Verification items for the finished model (mm, model axes). A direction names the side the tool comes from. Give positions to 0.01 mm unless a question says otherwise; leave off trailing zeros. Write each loop counter-clockwise with the first axis right and the second up, starting at its lowest first coordinate (ties: lowest second). Pieces come first, ordered by that corner, then holes. Notation, with made-up numbers: (-25, 81.5) -> (-9, 81.5) arc R16 cw to (-9, 106.5) -> close; hole circle Ø9 at (28, 69.25). An arc over 180 degrees is marked (long way). Write item = value, one per line.
from build123d import *

# Parameters (mm, degrees)
SKETCH1_W           = 215
SKETCH1_H           = 88
SKETCH1_R           = 1.75
BOSS_EXTRUDE1_DEPTH = 4
FILLET1_R           = 15
FILLET2_R           = 40
BOSS_EXTRUDE2_DEPTH = 160
SKETCH3_R           = 1.6
CUT_EXTRUDE1_DEPTH  = 4


with BuildPart() as part:
    # Sketch1 → Boss-Extrude1 (new body)
    with BuildSketch(Plane.XY):
        with Locations((-8, 0)):
            Rectangle(SKETCH1_W, SKETCH1_H)
        with Locations((-26.5, 20)):
            Circle(SKETCH1_R, mode=Mode.SUBTRACT)
        with Locations((26.5, 20)):
            Circle(SKETCH1_R, mode=Mode.SUBTRACT)
        with Locations((-26.5, -20)):
            Circle(SKETCH1_R, mode=Mode.SUBTRACT)
        with Locations((26.5, -20)):
            Circle(SKETCH1_R, mode=Mode.SUBTRACT)
        with Locations((0, 20)):
            Circle(SKETCH1_R, mode=Mode.SUBTRACT)
        with Locations((0, -20)):
            Circle(SKETCH1_R, mode=Mode.SUBTRACT)
    extrude(amount=BOSS_EXTRUDE1_DEPTH)

    # Fillet1
    fillet1_edges = [part.edges().sort_by_distance(p)[0] for p in [
        (99.5, -44, 2),
        (99.5, 44, 2),
    ]]
    fillet(fillet1_edges, radius=FILLET1_R)

    # Fillet2
    fillet2_edges = [part.edges().sort_by_distance(p)[0] for p in [
        (-115.5, -44, 2),
        (-115.5, 44, 2),
    ]]
    fillet(fillet2_edges, radius=FILLET2_R)

    # Sketch2 → Boss-Extrude2 (add)
    with BuildSketch(Plane.ZY.offset(75.5)):
        with BuildLine():
            Line((0, -44), (4, -44))
            ThreePointArc((4, -44), (4.439339828, -45.060660172), (5.5, -45.5))
            Line((5.5, -45.5), (16, -45.5))
            Line((16, -45.5), (16, -49.5))
            Line((16, -49.5), (5.5, -49.5))
            ThreePointArc((5.5, -49.5), (1.610912703, -47.889087297), (0, -44))
        make_face()
        with BuildLine():
            Line((16, 49.5), (5.5, 49.5))
            ThreePointArc((5.5, 49.5), (1.610912703, 47.889087297), (0, 44))
            Line((0, 44), (4, 44))
            ThreePointArc((4, 44), (4.439339828, 45.060660172), (5.5, 45.5))
            Line((5.5, 45.5), (16, 45.5))
            Line((16, 45.5), (16, 49.5))
        make_face()
    extrude(amount=-BOSS_EXTRUDE2_DEPTH)

    # Sketch3 → Cut-Extrude1 (cut)
    with BuildSketch(Plane.XY.offset(4)):
        with Locations((63.5, -32)):
            Circle(SKETCH3_R)
        with Locations((39.5, -32)):
            Circle(SKETCH3_R)
        with Locations((15.5, -32)):
            Circle(SKETCH3_R)
        with Locations((87.5, -32)):
            Circle(SKETCH3_R)
        with Locations((87.5, -16)):
            Circle(SKETCH3_R)
        with Locations((-8.5, -32)):
            Circle(SKETCH3_R)
        with Locations((-32.5, -32)):
            Circle(SKETCH3_R)
        with Locations((-56.5, -32)):
            Circle(SKETCH3_R)
        with Locations((-80.5, -32)):
            Circle(SKETCH3_R)
        with Locations((87.5, 0)):
            Circle(SKETCH3_R)
        with Locations((63.5, -16)):
            Circle(SKETCH3_R)
        with Locations((63.5, 0)):
            Circle(SKETCH3_R)
        with Locations((-56.5, -16)):
            Circle(SKETCH3_R)
        with Locations((-80.5, -16)):
            Circle(SKETCH3_R)
        with Locations((-104.5, -16)):
            Circle(SKETCH3_R)
        with Locations((-56.5, 0)):
            Circle(SKETCH3_R)
        with Locations((-80.5, 0)):
            Circle(SKETCH3_R)
        with Locations((-104.5, 0)):
            Circle(SKETCH3_R)
    cut_extrude1 = extrude(amount=-CUT_EXTRUDE1_DEPTH, mode=Mode.SUBTRACT)

    # Mirror5: Cut-Extrude1 across plane
    add(cut_extrude1.mirror(Plane.ZX), mode=Mode.SUBTRACT)


solid = part.part
Item 1: Sectioned sample at A-A on x = 69. Record the cut outline in (y, z).
Response values:
outline = (-49.5, 5.5) arc R5.5 ccw to (-44, 0) -> (44, 0) arc R5.5 ccw to (49.5, 5.5) -> (49.5, 16) -> (45.5, 16) -> (45.5, 5.5) arc R1.5 cw to (44, 4) -> (-44, 4) arc R1.5 cw to (-45.5, 5.5) -> (-45.5, 16) -> (-49.5, 16) -> close
Item 2: Go/stop test with flat-tipped pins: P1, Ø2.5, axis at x = -80.5, y = 32, coming from the -Z side; P2, Ø5, axis at x = -56.5, y = 32, coming from the +Z side; P3, Ø4, axis at x = 26.5, y = 20, coming from the -Z side. Record where each tip stops, or that it passes through.
Response values:
P1 = through
P2 = 4
P3 = 0
Item 3: Sectioned sample at C-C on x = -100. Record the cut outline in (y, z).
Response values:
outline = (-35.62, 0) -> (35.62, 0) -> (35.62, 4) -> (-35.62, 4) -> close
Item 4: Mould release check, pull along Y, two halves, no side actions. Record for faces 1 (the flat face through (84.5, 47, 8)), 2 (the cylindrical face through (3.38, 47.93, 1.65)), 3 (the flat face through (3, -45.5, 11)), 4 (the cylindrical face through (-103.472, -32.594, 2.028)): +Y half, -Y half, draft (parallel to the pull), parting line (faces both ways), or undercut.
Response values:
face_1 = draft
face_2 = +Y half
face_3 = undercut
face_4 = -Y half
Item 5: Sectioned sample at B-B on y = 38.5. Record the cut outline in (x, z).
Response values:
outline = (-95.74, 0) -> (96.11, 0) -> (96.11, 4) -> (-95.74, 4) -> close
Item 6: Set-up check for faces 5 (the flat face through (-75.5, -47, 8)), 6 (the flat face through (3, 45.5, 11)), 7 (the flat face through (-75.5, 47, 8)), 8 (the flat face through (84.5, -47, 8)): record each of +Z, -Z, +X, -X, +Y, -Y from which the full face is reachable in a straight line by a thin tool's end or side.
Response values:
face_5 = +Z, -Z, -X, -Y
face_6 = +Z, +X, -X
face_7 = +Z, -Z, -X, +Y
face_8 = +Z, -Z, +X, -Y
Item 7: Material ranges on line 1 (Y direction, x = -14.5, z = 5.5); line 2 (X direction, y = -1, z = 1.5); line 3 (Y direction, x = 15.5, z = 0.85), recorded low to high.
Response values:
line_1 = -49.5 to -45.5, 45.5 to 49.5
line_2 = -115.5 to -105.75, -103.25 to -81.75, -79.25 to -57.75, -55.25 to 62.25, 64.75 to 86.25, 88.75 to 99.5
line_3 = -46.94 to -33.6, -30.4 to 30.4, 33.6 to 46.94
